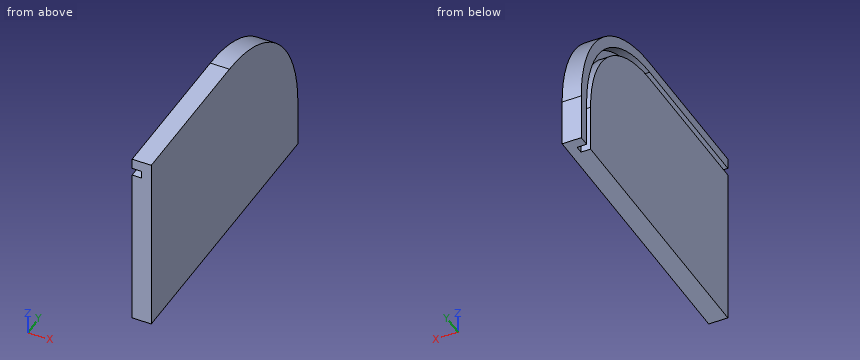
```python
from build123d import *

# Parameters (mm, degrees)
F0_W     = 300
F0_H     = 190
F1_DEPTH = 20
F2_R     = 140
F4_DEPTH = 10


with BuildPart() as f1:
    # F0 (on Right) → F1 (new body)
    with BuildSketch(Plane.YZ):
        Rectangle(F0_W, F0_H)
    extrude(amount=F1_DEPTH)

    # F2
    f2_edges = [f1.edges().sort_by_distance(p)[0] for p in [
        (10, 150, 95),
    ]]
    fillet(f2_edges, radius=F2_R)

    # F3 (on face) → F4 (cut)
    with BuildSketch(Plane(origin=(0, 0, 0), x_dir=(0, -1, 0), z_dir=(-1, 0, 0))):
        with BuildLine():
            Line((-139, -45), (-139, -95))
            Line((-139, -95), (-131, -95))
            Line((-131, -95), (-131, -45))
            ThreePointArc((-131, -45), (-95.559921, 40.559921), (-10, 76))
            Line((-10, 76), (150, 76))
            Line((150, 76), (150, 84))
            Line((150, 84), (-10, 84))
            ThreePointArc((-10, 84), (-101.216775, 46.216775), (-139, -45))
        make_face()
    extrude(amount=-F4_DEPTH, mode=Mode.SUBTRACT)


solid = f1.part
```
Geometry: final body of the model. Coordinates: model frame, mm. Round coordinates to 2 decimals unless told otherwise and drop trailing zeros. Order: outer loops, then holes, each group sorted by start corner. A loop starts at its lowest first (then second) coordinate and runs counter-clockwise, first axis right, second up. Notation, with made-up numbers: (89.25, 3.5) -> (122.25, 3.5) arc R22 ccw to (122.25, 18.5) -> close; hole circle Ø9 at (63, -39.5). An arc over 180 degrees is marked (long way). Use one line per item in the form item = value. Start each with the question number.
1. Pin query (flat end, axial travel): pin 1 Ø3 at (x, y) = (12.5, 91.5) entering from +Z; pin 2 Ø1 at (x, y) = (3.5, 105) entering from +Z. Return the tip coordinate at first contact, or that it passes through.
2. Cut plane B-B (y = -80.5). Return the cut outline in (x, z).
3. Line query: probe 1 along Z at (x, y) = (4.25, -116); probe 2 along Y at (x, z) = (7.5, -68); probe 3 along Z at (x, y) = (2, 74.5). Output: solid intervals per line, ascending.
4. Cut plane C-C (z = 66). Return the cut outline in (x, y).
5. Cut plane A-A (x = 5.5). Return the cut outline in (y, z).
Solution:
q1.pin_1 = 69.89
q1.pin_2 = 58.29
q2.outline = (0, -95) -> (20, -95) -> (20, 95) -> (0, 95) -> (0, 84) -> (10, 84) -> (10, 76) -> (0, 76) -> close
q3.probe_1 = -95 to 76, 84 to 95
q3.probe_2 = -150 to 131, 139 to 150
q3.probe_3 = -95 to 57.38, 66.72 to 79.26
q4.outline = (0, -150) -> (20, -150) -> (20, 95.32) -> (0, 95.32) -> (0, 75.73) -> (10, 75.73) -> (10, 58.17) -> (0, 58.17) -> close
q5.outline = (-150, -95) -> (131, -95) -> (131, -45) arc R121 ccw to (10, 76) -> (-150, 76) -> close; (-150, 84) -> (10, 84) arc R129 cw to (139, -45) -> (139, -95) -> (150, -95) -> (150, -45) arc R140 ccw to (10, 95) -> (-150, 95) -> close
